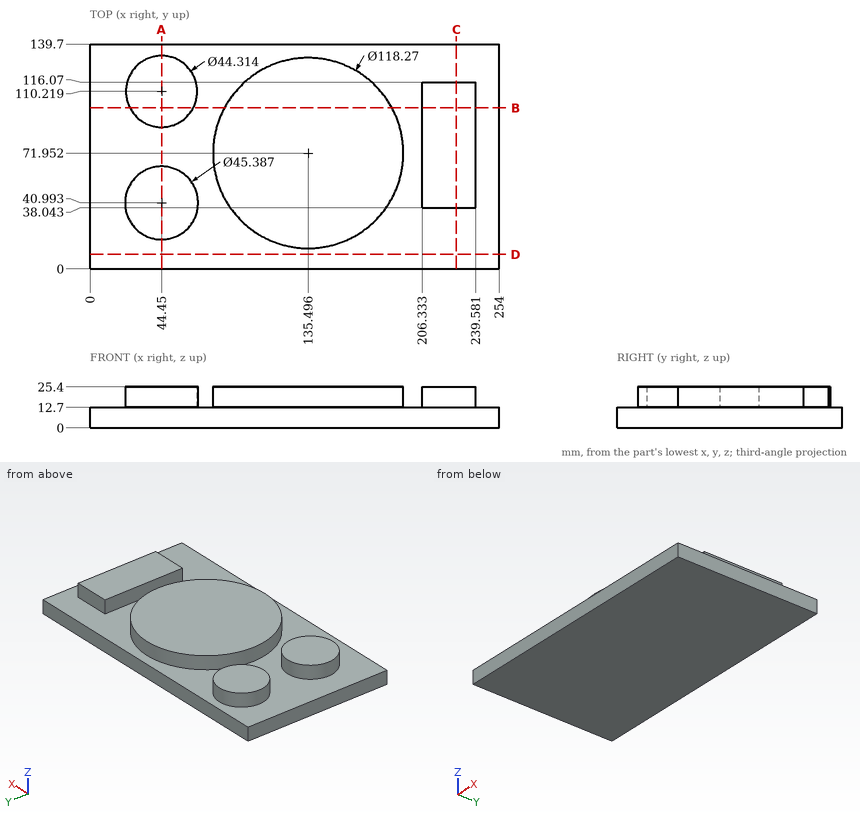
Job drawing, mm, ordinate dimensions from the low corner. One solid piece. Coordinates: 2 decimals unless noted, no trailing zeros. Write each loop counter-clockwise with the first axis right and the second up, starting at its lowest first coordinate (ties: lowest second). Pieces come first, ordered by that corner, then holes. Notation, with made-up numbers: M 63.5,8.5 L 98.5,8.5 A20 ccw 98.5,36.5 Z; hole C 25.5,0 d11. An arc over 180 degrees is marked long. Answer as a JSON object with one key per item and string values. Group by question number.
1) Saw through at A-A (x = 44.45). Write the cut outline in (y, z) (1 decimal), plus the area to 3 significant figures.
2) Pin check, flat tips, straight feed: pin 1 Ø6.5 at (y, z) = (80, 16.5) entering from +X; pin 2 Ø14 at (y, z) = (74.5, 20.5) entering from -X; pin 3 Ø10 at (x, z) = (225.5, 21) entering from +Y. Stop position of each tip, or through.
3) Saw through at D-D (y = 9). Write the cut outline in (x, z).
4) Saw through at B-B (y = 100). Write the cut outline in (x, z) (1 decimal), plus the area to 3 significant figures.
5) Wall check: line 1 (X direction, y = 48.5, z = 21) (1 decimal); line 2 (X direction, y = 107, z = 23) (1 decimal); line 3 (Z direction, x = 21.5, y = 40.5). Give the ranges that are in metal, low to high. Write a range as from..to.
6) Saw through at C-C (x = 227.5). Write the cut outline in (y, z), plus the area to 4 significant figures.
Values follow:
{
 "1": {"outline": "M 0,0 L 139.7,0 L 139.7,12.7 L 132.4,12.7 L 132.4,25.4 L 88.1,25.4 L 88.1,12.7 L 63.7,12.7 L 63.7,25.4 L 18.3,25.4 L 18.3,12.7 L 0,12.7 Z", "area": "2,910 mm2"},
 "2": {"pin 1": "stops at x = 239.58", "pin 2": "stops at x = 76.36", "pin 3": "stops at y = 116.07"},
 "3": {"outline": "M 0,0 L 254,0 L 254,12.7 L 0,12.7 Z"},
 "4": {"outline": "M 0,0 L 254,0 L 254,12.7 L 239.6,12.7 L 239.6,25.4 L 206.3,25.4 L 206.3,12.7 L 187.6,12.7 L 187.6,25.4 L 83.4,25.4 L 83.4,12.7 L 64.1,12.7 L 64.1,25.4 L 24.8,25.4 L 24.8,12.7 L 0,12.7 Z", "area": "5,470 mm2"},
 "5": {"line 1": "x = 23..65.9, 81.2..189.8, 206.3..239.6", "line 2": "x = 22.5..66.4, 87.9..183.1, 206.3..239.6", "line 3": "z = 0..12.7"},
 "6": {"outline": "M 0,0 L 139.7,0 L 139.7,12.7 L 116.07,12.7 L 116.07,25.4 L 38.04,25.4 L 38.04,12.7 L 0,12.7 Z", "area": "2,765 mm2"}
}
